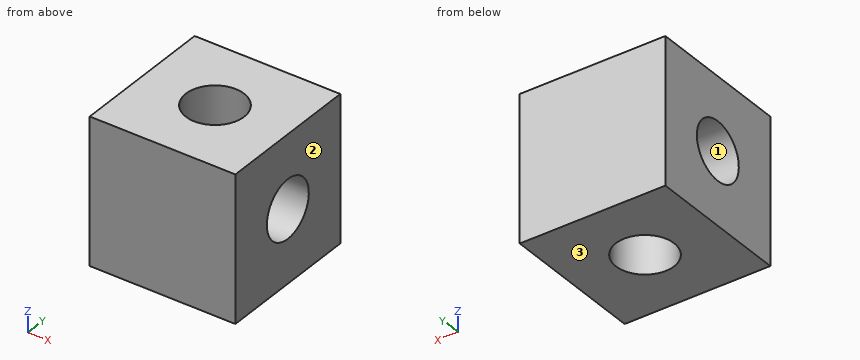
```python
from build123d import *

# Parameters (mm, degrees)
SKETCH_1_W          = 10
SKETCH_1_H          = 10
SKETCH_1_R          = 2
EXTRUDE_1_DEPTH     = 10
SKETCH_2_R          = 2
CUT_EXTRUDE_1_DEPTH = 16


with BuildPart() as part:
    # 草图1 → 凸台-拉伸1 (new body)
    with BuildSketch(Plane(origin=(0, 0, 0), x_dir=(0, 0, -1), z_dir=(1, 0, 0))):
        Rectangle(SKETCH_1_W, SKETCH_1_H)
        Circle(SKETCH_1_R, mode=Mode.SUBTRACT)
    extrude(amount=EXTRUDE_1_DEPTH)

    # 草图2 → 切除-拉伸1 (cut, through all)
    with BuildSketch(Plane(origin=(0, 0, -5), x_dir=(-1, 0, 0), z_dir=(0, 0, -1))):
        with Locations((-5, 0)):
            Circle(SKETCH_2_R)
    extrude(amount=-CUT_EXTRUDE_1_DEPTH, mode=Mode.SUBTRACT)


solid = part.part
```
Geometry check sheet. Reference: the model listing, model coordinates, mm. Face numbers are marked on the shaded views. Give positions to 0.01 mm unless a question says otherwise; leave off trailing zeros. Loops run counter-clockwise (first coordinate to the right, second up) from the corner with the lowest first, then second, coordinate; pieces in that order, holes last. Notation, with made-up numbers: M -5.5,-2.75 L 22.5,-2.75 A30 ccw 22.5,29.25 Z; hole C 19,67.25 d8. An arc over 180 degrees is marked long. Write item = value, one per line. Start each with the question number.
1. Section check D-D, the plane z = 4. Enter the section's corners in (x, y), plus the area to 3 significant figures.
2. Section check A-A, the plane y = 0. Enter the section's corners in (x, z), plus the area to 3 significant figures.
3. Section check C-C, the plane z = 1. Enter the section's corners in (x, y), plus the area to 3 significant figures.
4. Go/stop test with a flat-tipped pin: P1, Ø3, axis at y = 0, z = 0, coming from the +X side. Record where the tip stops, or that it passes through.
5. Thickness scan on probe 1 along Z at (x, y) = (1.9, 0); probe 2 along X at (y, z) = (0, -2.85). Record the ranges inside material, lowest first.
6. Section check B-B, the plane x = 4.75. Enter the section's corners in (y, z), plus the area to 3 significant figures.
7. Draft check along Z on the marked faces 1, 2 and 3. Enter one of: +Z half, -Z half, draft (parallel to the pull), parting line (faces both ways), or undercut.
Values follow:
q1.outline = M 0,-5 L 10,-5 L 10,5 L 0,5 Z; hole C 5,0 d4
q1.area = 87.4 mm^2
q2.outline = M 0,-5 L 3,-5 L 3,-2 L 0,-2 Z; M 0,2 L 3,2 L 3,5 L 0,5 Z; M 7,-5 L 10,-5 L 10,-2 L 7,-2 Z; M 7,2 L 10,2 L 10,5 L 7,5 Z
q2.area = 36.0 mm^2
q3.outline = M 0,-5 L 10,-5 L 10,-1.73 L 6,-1.73 A2 cw 4,-1.73 L 0,-1.73 Z; M 0,1.73 L 4,1.73 A2 cw 6,1.73 L 10,1.73 L 10,5 L 0,5 Z
q3.area = 64.6 mm^2
q4.P1 = through
q5.probe_1 = -5 to -2, 2 to 5
q5.probe_2 = 0 to 3, 7 to 10
q6.outline = M -5,-5 L -1.98,-5 L -1.98,-0.25 A2 cw -1.98,0.25 L -1.98,5 L -5,5 Z; M 1.98,-5 L 5,-5 L 5,5 L 1.98,5 L 1.98,0.25 A2 cw 1.98,-0.25 Z
q6.area = 60.3 mm^2
q7.face_1 = undercut
q7.face_2 = draft
q7.face_3 = -Z half
